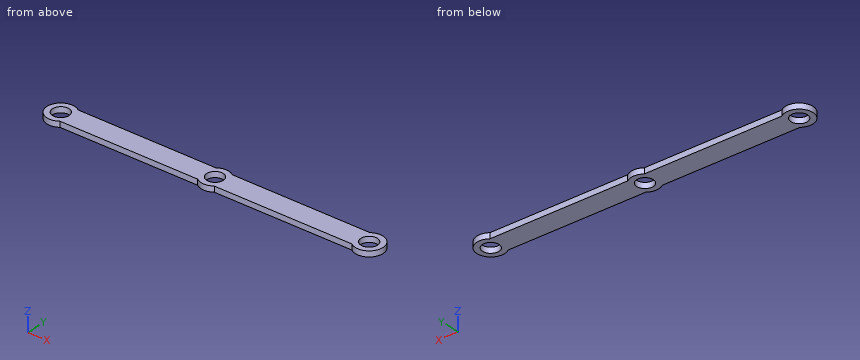
from build123d import *

# Parameters (mm, degrees)
SKETCH_1_R      = 1.5
EXTRUDE_1_DEPTH = 1


with BuildPart() as part:
    # 草图1 → 凸台-拉伸1 (new body)
    with BuildSketch(Plane.XY):
        with BuildLine():
            Line((1.5, 2), (26.5, 2))
            ThreePointArc((26.5, 2), (30.5, 0), (26.5, -2))
            Line((26.5, -2), (1.5, -2))
            ThreePointArc((1.5, -2), (0, -2.5), (-1.5, -2))
            Line((-1.5, -2), (-26.5, -2))
            ThreePointArc((-26.5, -2), (-30.5, 0), (-26.5, 2))
            Line((-26.5, 2), (-1.5, 2))
            ThreePointArc((-1.5, 2), (0, 2.5), (1.5, 2))
        make_face()
        with Locations((-28, 0)):
            Circle(SKETCH_1_R, mode=Mode.SUBTRACT)
        Circle(SKETCH_1_R, mode=Mode.SUBTRACT)
        with Locations((28, 0)):
            Circle(SKETCH_1_R, mode=Mode.SUBTRACT)
    extrude(amount=EXTRUDE_1_DEPTH)


solid = part.part
Part model, mm, in its own coordinate system. Coordinates: 2 decimals unless noted, no trailing zeros. Loops run counter-clockwise (first coordinate to the right, second up) from the corner with the lowest first, then second, coordinate; pieces in that order, holes last. Notation, with made-up numbers: M 30.25,74 L 80.25,74 A23 cw 80.25,90 Z; hole C 52,-9 d9. An arc over 180 degrees is marked long. Use a Markdown table: item, result. Add a question column.
Q1. Cut at C-C (y = 0). Write the cut outline in (x, z), and give its area (3 significant figures).
Q2. Pin check, flat tip, straight feed: P1, Ø2.5, axis at x = 0, y = 0, coming from the +Z side. Stop position of the tip, or through.
Q3. Cut at D-D (x = -8.5). Write the cut outline in (y, z), and give its area (3 significant figures).
Q4. Cut at B-B (z = 0.35). Write the cut outline in (x, y), and give its area (3 significant figures).
Q5. Probe L1, parallel to X at y = -2.1, z = 0.4; L2, parallel to Y at x = -28, z = 0.35; L3, parallel to X at y = 0.9, z = 0.5. List the from-to ranges inside material, lowest first.
Q6. Cut at A-A (x = 0). Write the cut outline in (y, z), and give its area (3 significant figures).
Worked out:
| question | item | result |
|---|---|---|
| 1 | outline | M -30.5,0 L -29.5,0 L -29.5,1 L -30.5,1 Z; M -26.5,0 L -1.5,0 L -1.5,1 L -26.5,1 Z; M 1.5,0 L 26.5,0 L 26.5,1 L 1.5,1 Z; M 29.5,0 L 30.5,0 L 30.5,1 L 29.5,1 Z |
| 1 | area | 52.0 mm2 |
| 2 | P1 | passes through |
| 3 | outline | M -2,0 L 2,0 L 2,1 L -2,1 Z |
| 3 | area | 4.00 mm2 |
| 4 | outline | M -26.5,-2 L -1.5,-2 A2.5 ccw 1.5,-2 L 26.5,-2 A2.5 ccw long 26.5,2 L 1.5,2 A2.5 ccw -1.5,2 L -26.5,2 A2.5 ccw long Z; hole C -28,0 d3; hole C 0,0 d3; hole C 28,0 d3 |
| 4 | area | 227 mm2 |
| 5 | L1 | x = -29.36 to -26.64, -1.36 to 1.36, 26.64 to 29.36 |
| 5 | L2 | y = -2.5 to -1.5, 1.5 to 2.5 |
| 5 | L3 | x = -30.33 to -29.2, -26.8 to -1.2, 1.2 to 26.8, 29.2 to 30.33 |
| 6 | outline | M -2.5,0 L -1.5,0 L -1.5,1 L -2.5,1 Z; M 1.5,0 L 2.5,0 L 2.5,1 L 1.5,1 Z |
| 6 | area | 2.00 mm2 |
